For this review, take the finished solid that the model builds, in its own axes (mm). A direction names the side the tool comes from. Coordinates: 2 decimals unless noted, no trailing zeros. Loops run counter-clockwise (first coordinate to the right, second up) from the corner with the lowest first, then second, coordinate; pieces in that order, holes last. Notation, with made-up numbers: M -20.75,53 L -4.75,53 A29 cw -4.75,84 Z; hole C 44.5,0 d9. An arc over 180 degrees is marked long. Answer as a JSON object with one key per item and string values. Group by question number.
Item 1: Add section A-A (x = 201). State the section outline as (y, z) points, then the cut area to 3 significant figures.
Item 2: Add section B-B (z = -659). State the section outline as (x, y) points.
Item 3: Wall thickness on L1, parallel to X at y = 34.5, z = -47; L2, parallel to Z at x = 103, y = 22: over which ranges is each line inside the solid? List them lowest first. Write a range as from..to.
Item 4: Mouldability with a two-part tool opening along X and no side actions: class faces 3 (the face through (233, 20, -973.726)), 4 (the face through (512.034, 20, -467)), 5 (the face through (233, 20, -943.726)), 6 (the face through (-67.966, 20, -467)) as +X half, -X half, draft (parallel to the pull), parting line (faces both ways), or undercut.
Item 5: Tool access review of faces 1 (the face through (-37.966, 20, -467)), 2 (the face through (542.034, 20, -467)): name each direction out of +Z, -Z, +X, -X, +Y, -Y from which nothing blocks a thin tool from reaching the whole face with its end or side.
from build123d import *

# Parameters (mm, degrees)
SKETCH_1_W          = 610
SKETCH_1_H          = 1000
SKETCH_1_W_2        = 550
SKETCH_1_H_2        = 940
EXTRUDE_1_DEPTH     = 40
SKETCH_2_R          = 5
CUT_EXTRUDE_1_DEPTH = 611


with BuildPart() as part:
    # Эскиз1 → Бобышка-Вытянуть1 (new body)
    with BuildSketch(Plane(origin=(0, 0, 0), x_dir=(1, 0, 0), z_dir=(0, 1, 0))):
        with Locations((237.034264066, 473.725626833)):
            Rectangle(SKETCH_1_W, SKETCH_1_H)
        with Locations((237.034264066, 473.725626833)):
            Rectangle(SKETCH_1_W_2, SKETCH_1_H_2, mode=Mode.SUBTRACT)
    extrude(amount=EXTRUDE_1_DEPTH)

    # Эскиз2 → Вырез-Вытянуть1 (cut, through all)
    with BuildSketch(Plane(origin=(542.034264066, 0, 0), x_dir=(0, 0, -1), z_dir=(1, 0, 0))):
        with Locations((633.725626833, 20)):
            Circle(SKETCH_2_R)
    extrude(amount=-CUT_EXTRUDE_1_DEPTH, mode=Mode.SUBTRACT)


solid = part.part
From the geometry:
{
 "1": {"outline": "M 0,-973.73 L 40,-973.73 L 40,-943.73 L 0,-943.73 Z; M 0,-3.73 L 40,-3.73 L 40,26.27 L 0,26.27 Z", "area": "2,400 mm²"},
 "2": {"outline": "M -67.97,0 L -37.97,0 L -37.97,40 L -67.97,40 Z; M 512.03,0 L 542.03,0 L 542.03,40 L 512.03,40 Z"},
 "3": {"L1": "x = -67.97..-37.97, 512.03..542.03", "L2": "z = -973.73..-943.73, -3.73..26.27"},
 "4": {"face 3": "draft", "face 4": "undercut", "face 5": "undercut", "face 6": "-X half"},
 "5": {"face 1": "+Y, -Y", "face 2": "+Z, -Z, +X, +Y, -Y"}
}
